Source: CAD feature listing. Evaluate the final solid. Frame: model axes, mm. A direction names the side the tool comes from. Give positions to 0.01 mm unless a question says otherwise; leave off trailing zeros. Loops run counter-clockwise (first coordinate to the right, second up) from the corner with the lowest first, then second, coordinate; pieces in that order, holes last. Notation, with made-up numbers: (8.25, -19.5) -> (32.25, -19.5) arc R23 ccw to (32.25, -10.5) -> close; hole circle Ø11 at (29.25, 62.5). An arc over 180 degrees is marked (long way). Put each result on its own line as item: value.
```python
from build123d import *

# Parameters (mm, degrees)
SKETCH1_W           = 75
SKETCH1_H           = 45
BOSS_EXTRUDE1_DEPTH = 3.5
SKETCH2_W           = 74.999337444
SKETCH2_H           = 100
BOSS_EXTRUDE2_DEPTH = 3.5
SKETCH3_R           = 8
SKETCH3_R_2         = 2.5
CUT_EXTRUDE2_DEPTH  = 132.48954331


with BuildPart() as part:
    # Sketch1 → Boss-Extrude1 (new body)
    with BuildSketch(Plane(origin=(0, 0, 0), x_dir=(1, 0, 0), z_dir=(0, 1, 0))):
        with Locations((37.5, 22.5)):
            Rectangle(SKETCH1_W, SKETCH1_H)
    extrude(amount=BOSS_EXTRUDE1_DEPTH)

    # Sketch2 → Boss-Extrude2 (add)
    with BuildSketch(Plane(origin=(0, 0, -45), x_dir=(-1, 0, 0), z_dir=(0, 0, -1))):
        with Locations((-37.499668722, -46.5)):
            Rectangle(SKETCH2_W, SKETCH2_H)
    extrude(amount=BOSS_EXTRUDE2_DEPTH)

    # Sketch3 → Cut-Extrude2 (cut, through all)
    with BuildSketch(Plane(origin=(0, 0, -48.5), x_dir=(-1, 0, 0), z_dir=(0, 0, -1))):
        with Locations((-37.49990734, -24.47055223)):
            Circle(SKETCH3_R)
        with Locations((-37.49990734, -72.02944777)):
            Circle(SKETCH3_R)
        with Locations((-37.499668722, -48.25)):
            Circle(SKETCH3_R_2)
    extrude(amount=-CUT_EXTRUDE2_DEPTH, mode=Mode.SUBTRACT)


solid = part.part
```
(1) Section B-B on x = 43. Return loops of the section in (y, z).
Calculated:
outline: (-96.5, -48.5) -> (-77.84, -48.5) -> (-77.84, -45) -> (-96.5, -45) -> close; (-66.22, -48.5) -> (-30.28, -48.5) -> (-30.28, -45) -> (-66.22, -45) -> close; (-18.66, -48.5) -> (3.5, -48.5) -> (3.5, 0) -> (0, 0) -> (0, -45) -> (-18.66, -45) -> close
(2) Section D-D on z = -29.5. Return loops of the section in (x, y), then the cut area to 4 significant figures.
Calculated:
outline: (0, 0) -> (75, 0) -> (75, 3.5) -> (0, 3.5) -> close
area: 262.5 mm²
(3) Section C-C on x = 10.5. Return loops of the section in (y, z), then the cut area to 4 significant figures.
Calculated:
outline: (-96.5, -48.5) -> (3.5, -48.5) -> (3.5, 0) -> (0, 0) -> (0, -45) -> (-96.5, -45) -> close
area: 507.5 mm²
(4) Line query: probe 1 along X at (y, z) = (-48, -46); probe 2 along Y at (x, z) = (18.5, -1.5); probe 3 along Z at (x, y) = (29.5, -64.5). Output: solid intervals per line, ascending. Write a range as from..to.
Calculated:
probe 1: x = 0..35.01, 39.99..75
probe 2: y = 0..3.5
probe 3: z = -48.5..-45
(5) Draft query along X for faces 3 (the flat face through (38, -96.5, -47)), 4 (the flat face through (75, 2, -22)), 5 (the flat face through (0, -32, -46)), 6 (the cylindrical face through (45.492, -24.119, -46.774)). Return one class per face: released by +X, released by -X, zero draft, split by the parting line, or undercut.
Calculated:
face 3: zero draft
face 4: released by +X
face 5: released by -X
face 6: undercut
(6) First-contact query: P1, Ø21, axis at x = 37.5, y = -72.03, coming from the -Z side; P2, Ø6, axis at x = 40, y = -22.5, coming from the +Z side; P3, Ø5, axis at x = 27.5, y = -51, coming from the +Z side; P4, Ø5, axis at x = 31.5, z = -23.5, coming from the -Y side. Flat tips, straight axial feed; report the tip coordinate or a pass-through.
Calculated:
P1: stops at z = -48.5
P2: passes through
P3: stops at z = -45
P4: stops at y = 0
(7) Reachability of faces 1 (the flat face through (37, 0, -23)), 2 (the flat face through (46, -46, -48.5)) from +Z, -Z, +X, -X, +Y, -Y: full face, straight path, thin tool, end or side. Return the list, or none.
Calculated:
face 1: +Z, +X, -X, -Y
face 2: -Z, +X, -X, +Y, -Y
(8) Section A-A on y = -48.25. Return loops of the section in (x, z).
Calculated:
outline: (0, -48.5) -> (35, -48.5) -> (35, -45) -> (0, -45) -> close; (40, -48.5) -> (75, -48.5) -> (75, -45) -> (40, -45) -> close
